For this review, take the finished solid that the model builds, in its own axes (mm). A direction names the side the tool comes from. Round coordinates to 2 decimals unless told otherwise and drop trailing zeros. Order: outer loops, then holes, each group sorted by start corner. A loop starts at its lowest first (then second) coordinate and runs counter-clockwise, first axis right, second up. Notation, with made-up numbers: (65.25, 1.25) -> (99.25, 1.25) arc R16 cw to (99.25, 27.25) -> close; hole circle Ø3 at (29, 60). An arc over 180 degrees is marked (long way). Put each result on its own line as item: value. Start each with the question number.
Autodesk Inventor part; units mm, degrees
ref_plane "YZ Plane" through (0, 0, 0) normal (1, 0, 0) x (0, 1, 0)
ref_plane "XZ Plane" through (0, 0, 0) normal (0, 1, 0) x (-1, 0, 0)
ref_plane "XY Plane" through (0, 0, 0) normal (0, 0, 1) x (1, 0, 0)
sketch "Sketch1" plane through (0, 0, 0) normal (0, 0, 1) x (1, 0, 0)
  circle A0 centre (0, 0) radius 50
  circle A1 centre (0, 0) radius 52
  dimension "d0" = 100
  dimension "d1" = 2
extrude "Extrusion1" add sketch "Sketch1" along normal blind 300
sketch "Sketch2" plane through (0, 0, 0) normal (0, 0, -1) x (-1, 0, 0)
  circle A0 centre (0, 0) radius 52
extrude "Extrusion2" add sketch "Sketch2" along normal blind 1
sketch "Sketch3" plane through (0, 0, 300) normal (0, 0, 1) x (1, 0, 0)
  circle A0 centre (0, 0) radius 52
extrude "Extrusion3" add sketch "Sketch3" along normal blind 1
properties part number "Chamber"
Item 1: Tool access review of faces 3 (the face through (1, 1, 0)), 4 (the face through (-1, 1, 301)): name each direction out of +Z, -Z, +X, -X, +Y, -Y from which nothing blocks a thin tool from reaching the whole face with its end or side.
Item 2: Consider section A-A, the plane x = 0. Write out the cut boundary in (y, z), plus the area to 3 significant figures.
Item 3: Insertion check: pin 1 Ø5 at (x, z) = (11, 164.5) entering from -Y; pin 2 Ø8 at (y, z) = (17.5, 64.5) entering from +X; pin 3 Ø1 at (x, z) = (-19, 110) entering from +Y. Each pin has a flat end and moves straight along its axis. Give the tip position at first contact, or say it passes through.
Item 4: For L1, parallel to Z at x = 48, y = -2.5; L2, parallel to Y at x = 0, z = 118; L3, parallel to Y at x = 3.5, z = 217.5, list the stretches that pass through material, from the lowest coordinate up.
Item 5: Consider section C-C, the plane z = 85. Write out the cut boundary in (x, y).
Item 6: Mouldability with a two-part tool opening along Y and no side actions: class faces 1 (the face through (-1, 1, 300)), 2 (the face through (1, 1, -1)) as +Y half, -Y half, draft (parallel to the pull), parting line (faces both ways), or undercut.
Evaluation:
1. face 3: none
1. face 4: +Z, +X, -X, +Y, -Y
2. outline: (-52, -1) -> (52, -1) -> (52, 301) -> (-52, 301) -> close; hole (-50, 0) -> (50, 0) -> (50, 300) -> (-50, 300) -> close
2. area: 1,410 mm^2
3. pin 1: stops at y = -51.3
3. pin 2: stops at x = 50.22
3. pin 3: stops at y = 48.6
4. L1: z = -1 to 0, 300 to 301
4. L2: y = -52 to -50, 50 to 52
4. L3: y = -51.88 to -49.88, 49.88 to 51.88
5. outline: circle Ø104 at (0, 0); hole circle Ø100 at (0, 0)
6. face 1: undercut
6. face 2: draft
